Autodesk Inventor part; units mm, degrees
ref_plane "YZ Plane" through (0, 0, 0) normal (1, 0, 0) x (0, 1, 0)
ref_plane "XZ Plane" through (0, 0, 0) normal (0, 1, 0) x (-1, 0, 0)
ref_plane "XY Plane" through (0, 0, 0) normal (0, 0, 1) x (1, 0, 0)
sketch "スケッチ1" plane through (0, 0, 0) normal (0, 0, 1) x (1, 0, 0)
  circle A0 centre (-12.7279, -12.7279) radius 6
  arc A1 (-11.767, -8.0827) -> (-12.7279, -7.5279) centre (-12.7279, -8.6375) ccw
  arc A2 (-12.7279, -7.5279) -> (-13.6889, -8.0827) centre (-12.7279, -8.6375) ccw
  arc A3 (-16.2703, -9.5731) -> (-13.6889, -8.0827) centre (-16.2703, -6.5923) ccw
  arc A4 (-16.2703, -9.5731) -> (-17.2313, -10.1279) centre (-16.2703, -10.6827) ccw
  arc A5 (-17.2313, -10.1279) -> (-17.2313, -11.2375) centre (-16.2703, -10.6827) ccw
  arc A6 (-17.2313, -14.2183) -> (-17.2313, -11.2375) centre (-19.8127, -12.7279) ccw
  arc A7 (-17.2313, -14.2183) -> (-17.2313, -15.3279) centre (-16.2703, -14.7731) ccw
  arc A8 (-17.2313, -15.3279) -> (-16.2703, -15.8827) centre (-16.2703, -14.7731) ccw
  arc A9 (-13.6889, -17.3731) -> (-16.2703, -15.8827) centre (-16.2703, -18.8635) ccw
  arc A10 (-13.6889, -17.3731) -> (-12.7279, -17.9279) centre (-12.7279, -16.8183) ccw
  arc A11 (-12.7279, -17.9279) -> (-11.767, -17.3731) centre (-12.7279, -16.8183) ccw
  arc A12 (-9.1855, -15.8827) -> (-11.767, -17.3731) centre (-9.1855, -18.8635) ccw
  arc A13 (-9.1855, -15.8827) -> (-8.2246, -15.3279) centre (-9.1855, -14.7731) ccw
  arc A14 (-8.2246, -15.3279) -> (-8.2246, -14.2183) centre (-9.1855, -14.7731) ccw
  arc A15 (-8.2246, -11.2375) -> (-8.2246, -14.2183) centre (-5.6431, -12.7279) ccw
  arc A16 (-8.2246, -11.2375) -> (-8.2246, -10.1279) centre (-9.1855, -10.6827) ccw
  arc A17 (-8.2246, -10.1279) -> (-9.1855, -9.5731) centre (-9.1855, -10.6827) ccw
  arc A18 (-11.767, -8.0827) -> (-9.1855, -9.5731) centre (-9.1855, -6.5923) ccw
  point P0 (0, 0)
  point P1 (0, 0)
extrude "押し出し1" add sketch "スケッチ1" along normal blind 5.5
sketch "書き出し" plane through (-12.7279, -12.7279, 5.5) normal (0, 0, 1) x (1, 0, 0)
  circle A0 centre (0, 0) radius 6
  arc A1 (4.5033, 1.4904) -> (4.5033, -1.4904) centre (7.0848, 0) ccw
  arc A2 (3.5424, -3.1548) -> (4.5033, -1.4904) centre (3.5424, -2.0452) ccw
  arc A3 (3.5424, -3.1548) -> (0.9609, -4.6452) centre (3.5424, -6.1356) ccw
  arc A4 (-0.9609, -4.6452) -> (0.9609, -4.6452) centre (0, -4.0904) ccw
  arc A5 (-0.9609, -4.6452) -> (-3.5424, -3.1548) centre (-3.5424, -6.1356) ccw
  arc A6 (-4.5033, -1.4904) -> (-3.5424, -3.1548) centre (-3.5424, -2.0452) ccw
  arc A7 (-4.5033, -1.4904) -> (-4.5033, 1.4904) centre (-7.0848, 0) ccw
  arc A8 (-3.5424, 3.1548) -> (-4.5033, 1.4904) centre (-3.5424, 2.0452) ccw
  arc A9 (-3.5424, 3.1548) -> (-0.9609, 4.6452) centre (-3.5424, 6.1356) ccw
  arc A10 (0.9609, 4.6452) -> (-0.9609, 4.6452) centre (0, 4.0904) ccw
  arc A11 (0.9609, 4.6452) -> (3.5424, 3.1548) centre (3.5424, 6.1356) ccw
  arc A12 (4.5033, 1.4904) -> (3.5424, 3.1548) centre (3.5424, 2.0452) ccw
  point P0 (12.7279, 12.7279)
properties part number "原動節接続部v2外" material "アルミニウム 2014-T4"
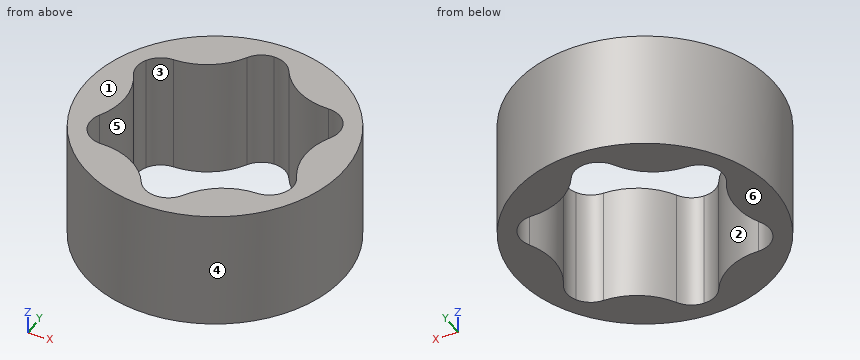
Can you work these out from the model? Positions are in its coordinate system, mm. Face numbers are marked on the shaded views. A direction names the side the tool comes from. Give positions to 0.01 mm unless a question says otherwise; leave off trailing zeros. Write each loop counter-clockwise with the first axis right and the second up, starting at its lowest first coordinate (ties: lowest second). Pieces come first, ordered by that corner, then holes. Notation, with made-up numbers: (42.25, 51.25) -> (56.25, 51.25) arc R20 cw to (56.25, 62.25) -> close; hole circle Ø9 at (10, -13). An arc over 180 degrees is marked (long way). Answer as a JSON object with one key per item and string values. Group by question number.
Item 1: Please list where these lines run through material, in increasing order: line 1 (X direction, y = -13, z = 0.35); line 2 (X direction, y = -12, z = 4.2); line 3 (Y direction, x = -11.5, z = 4.65). Write a range as [from, to].
Item 2: Suppose I cut it at D-D (x = -15.75). Please give me the cut outline in (y, z).
Item 3: I'm going to push flat-ended pins straight in: P1, Ø2, axis at y = -15, z = 4.5, coming from the -X side; P2, Ø3, axis at y = -16.5, z = 3, coming from the -X side; P3, Ø3, axis at x = -17.5, z = 3, coming from the -Y side. Where does each tip first touch, or does it pass through?
Item 4: We'd pull the mould along Y, two halves only. Please class the marked faces 1, 2, 3 and 4: +Y half, -Y half, draft (parallel to the pull), parting line (faces both ways), or undercut.
Item 5: Suppose I cut it at C-C (y = -14). Please give me the cut outline in (x, z), plus the area to 3 significant figures.
Item 6: Suppose I cut it at A-A (z = 1.4). Please give me the cut outline in (x, y).
Item 7: Suppose I cut it at B-B (x = -17). Please give me the cut outline in (y, z), plus the area to 3 significant figures.
Item 8: For the marked faces 5 and 6, which set-ups out of +Z, -Z, +X, -X, +Y, -Y let a thin tool reach every point of the face, with its end or its side?
Findings:
{
 "1": {"line 1": "x = [-18.72, -16.84], [-8.61, -6.73]", "line 2": "x = [-18.68, -16.92], [-8.53, -6.77]", "line 3": "y = [-18.6, -16.99], [-8.47, -6.85]"},
 "2": {"outline": "(-17.91, 0) -> (-15.93, 0) -> (-15.93, 5.5) -> (-17.91, 5.5) -> close; (-9.53, 0) -> (-7.54, 0) -> (-7.54, 5.5) -> (-9.53, 5.5) -> close"},
 "3": {"P1": "stops at x = -18.59", "P2": "stops at x = -18.28", "P3": "stops at y = -17.76"},
 "4": {"face 1": "draft", "face 2": "undercut", "face 3": "undercut", "face 4": "parting line"},
 "5": {"outline": "(-18.59, 0) -> (-17.12, 0) -> (-17.12, 5.5) -> (-18.59, 5.5) -> close; (-8.34, 0) -> (-6.86, 0) -> (-6.86, 5.5) -> (-8.34, 5.5) -> close", "area": "16.2 mm²"},
 "6": {"outline": "circle Ø12 at (-12.73, -12.73); hole (-17.23, -15.33) arc R1.11 ccw to (-16.27, -15.88) arc R2.98 cw to (-13.69, -17.37) arc R1.11 ccw to (-12.73, -17.93) arc R1.11 ccw to (-11.77, -17.37) arc R2.98 cw to (-9.19, -15.88) arc R1.11 ccw to (-8.22, -15.33) arc R1.11 ccw to (-8.22, -14.22) arc R2.98 cw to (-8.22, -11.24) arc R1.11 ccw to (-8.22, -10.13) arc R1.11 ccw to (-9.19, -9.57) arc R2.98 cw to (-11.77, -8.08) arc R1.11 ccw to (-12.73, -7.53) arc R1.11 ccw to (-13.69, -8.08) arc R2.98 cw to (-16.27, -9.57) arc R1.11 ccw to (-17.23, -10.13) arc R1.11 ccw to (-17.23, -11.24) arc R2.98 cw to (-17.23, -14.22) arc R1.11 ccw to start"},
 "7": {"outline": "(-16.94, 0) -> (-15.61, 0) -> (-15.61, 5.5) -> (-16.94, 5.5) -> close; (-13.71, 0) -> (-11.74, 0) -> (-11.74, 5.5) -> (-13.71, 5.5) -> close; (-9.85, 0) -> (-8.51, 0) -> (-8.51, 5.5) -> (-9.85, 5.5) -> close", "area": "25.5 mm²"},
 "8": {"face 5": "+Z, -Z", "face 6": "-Z, +X, -X, +Y, -Y"}
}
